The listing builds one solid part. Answer for the finished solid, in the listing's coordinates (mm). A direction names the side the tool comes from. Round coordinates to 2 decimals unless told otherwise and drop trailing zeros. Write each loop counter-clockwise with the first axis right and the second up, starting at its lowest first coordinate (ties: lowest second). Pieces come first, ordered by that corner, then holes.
(1) Find the intervals of material crossed by probe 1 along Y at (x, z) = (0, 6); probe 2 along Z at (x, y) = (692.5, -349); probe 3 along Y at (x, z) = (-20, -364), in increasing order.
(2) The mould has two halves that part along X. Classify faces 6 (the face through (-779.07, -450.61, -382.08)), 7 (the face through (699, 286, 25)), 8 (the face through (403.2, 632.4, 12.3)): +X half, -X half, draft (parallel to the pull), parting line (faces both ways), or undercut.
(3) A cutting plane is placed at D-D, the plane y = 305. Give the vertices of the cut face in (x, z), and give its area (3 significant figures).
(4) Each of these flat-tipped pins is pushed along its axis until it touches: pin 1 Ø5 at (x, z) = (-1, -514.5) entering from +Y; pin 2 Ø1 at (y, z) = (-490, -155.5) entering from -X; pin 3 Ø10 at (x, z) = (-708, -471) entering from -Y; pin 4 Ø10 at (x, y) = (-649.5, 364) entering from +Z. Where does it stop, or does it pass through?
(5) A cutting plane is placed at B-B, the plane z = -575. Give the vertices of the cut face in (x, y), and give its area (3 significant figures).
(6) For faces 1 (the face through (-1, 800, -382)), 2 (the face through (-693.17, -399.394, -382.075)), 3 (the face through (760.52, -381.35, -382.08)), 4 (the face through (780, -449, -382)), 5 (the face through (50, 851, -382)), determine the directions among +Z, -Z, +X, -X, +Y, -Y from which every point of the face is accessible in a straight line to the end or side of a thin tool.
(7) A cutting plane is placed at A-A, the plane x = 0. Give the vertices of the cut face in (y, z), and give its area (3 significant figures).
(8) A cutting plane is placed at C-C, the plane y = 0. Give the vertices of the cut face in (x, z), and give its area (3 significant figures).
from build123d import *

# Parameters (mm, degrees)
F0_R     = 950
F0_R_2   = 750
F1_DEPTH = 25
F2_W     = 100
F2_H     = 100
F3_DEPTH = 775


with BuildPart() as f1:
    # F0 (on Top) → F1 (new body)
    with BuildSketch(Plane.XY):
        Circle(F0_R)
        Circle(F0_R_2, mode=Mode.SUBTRACT)
    extrude(amount=F1_DEPTH)

    # F2 (on face) → F3 (join)
    with BuildSketch(Plane(origin=(0, 0, 0), x_dir=(1, 0, 0), z_dir=(0, 0, -1))):
        with Locations((0, -850)):
            Rectangle(F2_W, F2_H)
        Polygon((-717.820323, 356.69873), (-667.820323, 443.30127), (-754.422863, 493.30127), (-804.422863, 406.69873), align=None)
        Polygon((667.820323, 443.30127), (717.820323, 356.69873), (804.422863, 406.69873), (754.422863, 493.30127), align=None)
    extrude(amount=F3_DEPTH)


solid = f1.part
Solutions:
1. probe 1: y = -950 to -750, 750 to 950
1. probe 2: z = 0 to 25
1. probe 3: y = 800 to 900
2. face 6: -X half
2. face 7: draft
2. face 8: undercut
3. outline: (-899.71, 0) - (-685.18, 0) - (-685.18, 25) - (-899.71, 25) - close; (685.18, 0) - (899.71, 0) - (899.71, 25) - (685.18, 25) - close
3. area: 10,700 mm2
4. pin 1: stops at y = 900
4. pin 2: stops at x = -756.62
4. pin 3: stops at y = -469.39
4. pin 4: passes through
5. outline: (-804.42, -406.7) - (-754.42, -493.3) - (-667.82, -443.3) - (-717.82, -356.7) - close; (-50, 800) - (50, 800) - (50, 900) - (-50, 900) - close; (667.82, -443.3) - (754.42, -493.3) - (804.42, -406.7) - (717.82, -356.7) - close
5. area: 30,000 mm2
6. face 1: -Z, +X, -X, -Y
6. face 2: -Z, +Y
6. face 3: -Z, +X, +Y
6. face 4: -Z, +X, -Y
6. face 5: -Z, +X, +Y, -Y
7. outline: (-950, 0) - (-750, 0) - (-750, 25) - (-950, 25) - close; (750, 0) - (800, 0) - (800, -775) - (900, -775) - (900, 0) - (950, 0) - (950, 25) - (750, 25) - close
7. area: 87,500 mm2
8. outline: (-950, 0) - (-750, 0) - (-750, 25) - (-950, 25) - close; (750, 0) - (950, 0) - (950, 25) - (750, 25) - close
8. area: 10,000 mm2
